For this review, use the dimensioned drawing (mm, ordinates from the lowest corner) and the shaded views. Round coordinates to 2 decimals unless told otherwise and drop trailing zeros. Order: outer loops, then holes, each group sorted by start corner. A loop starts at its lowest first (then second) coordinate and runs counter-clockwise, first axis right, second up. Notation, with made-up numbers: M 19.5,11.5 L 57.5,11.5 A30 cw 57.5,38.5 Z; hole C 38.5,5.25 d5. An arc over 180 degrees is marked long. Use a Markdown table: item, result. Add a question column.
1. Insertion check: P1, Ø12, axis at x = 32, z = 11, coming from the -Y side; P2, Ø0.9, axis at y = 1.5, z = 35.5, coming from the +X side; P3, Ø1.5, axis at y = 2, z = 6.5, coming from the -X side; P4, Ø1.5, axis at x = 9.5, y = 2, coming from the -Z side. Each pin has a flat end and moves straight along its axis. Give the tip position at first contact, or say it passes through.
2. The part is to be moulded in two halves that separate along X. For the marked faces 1, 2 and 3, say which applies: +X half, -X half, draft (parallel to the pull), parting line (faces both ways), or undercut.
3. Consider section A-A on z = 20.75. State the section outline as (x, y) points.
4. Consider section B-B on x = 20.75. State the section outline as (y, z) points, then the cut area to 3 significant figures.
5. Consider section C-C on x = 3. State the section outline as (y, z) points, then the cut area to 3 significant figures.
6. Consider section D-D on y = 0.95. Count the separate pieces of the cut face and the enclosed holes in it, then the cut area to 3 significant figures.
7. To check wall thickness, follow probe 1 along X at (y, z) = (1.9, 20.75); probe 2 along Z at (x, y) = (20.75, 1.6); probe 3 along Z at (x, y) = (38, 1). State the ranges of each line that lie inside material, in increasing order.
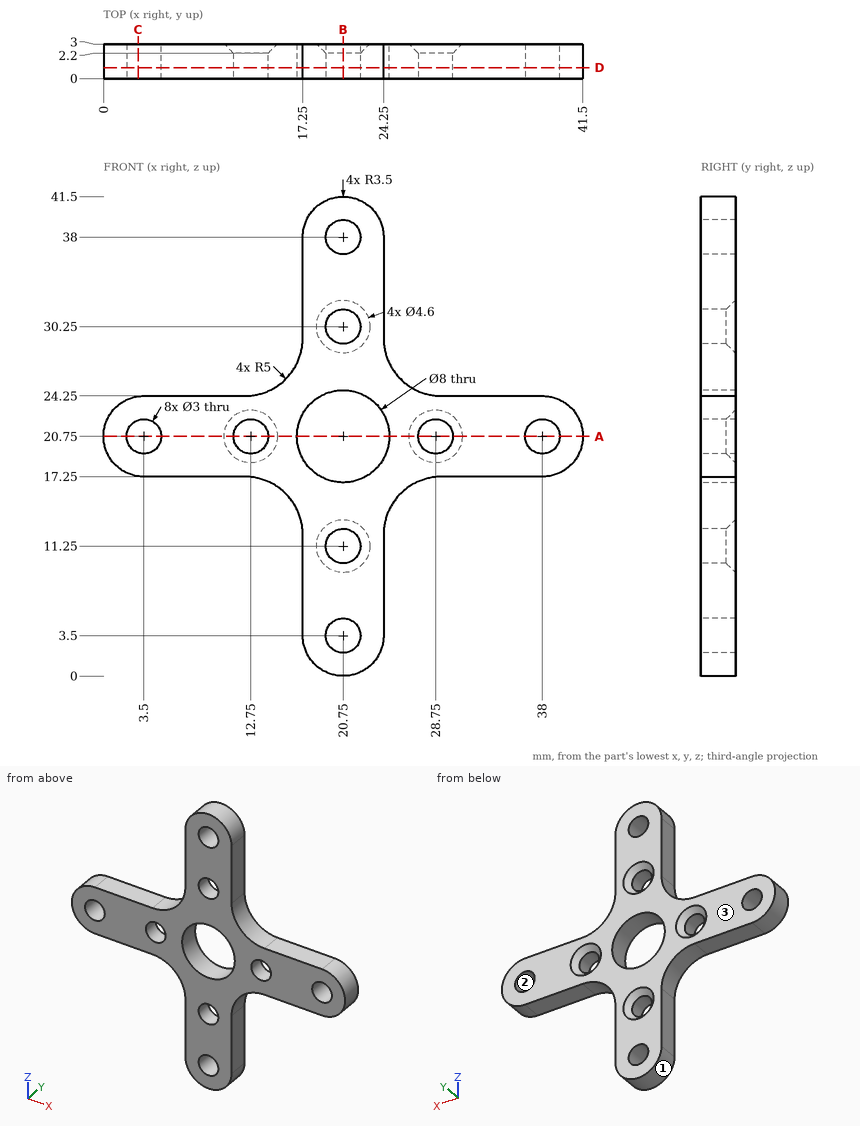
Answer block:
| question | item | result |
|---|---|---|
| 1 | P1 | through |
| 1 | P2 | x = 24.25 |
| 1 | P3 | x = 17.25 |
| 1 | P4 | z = 17.25 |
| 2 | face 1 | parting line |
| 2 | face 2 | undercut |
| 2 | face 3 | draft |
| 3 | outline | M 0,0 L 2,0 L 2,3 L 0,3 Z; M 5,0 L 11.25,0 L 11.25,2.2 L 10.45,3 L 5,3 Z; M 14.25,0 L 16.75,0 L 16.75,3 L 15.05,3 L 14.25,2.2 Z; M 24.75,0 L 27.25,0 L 27.25,2.2 L 26.45,3 L 24.75,3 Z; M 30.25,0 L 36.5,0 L 36.5,3 L 31.05,3 L 30.25,2.2 Z; M 39.5,0 L 41.5,0 L 41.5,3 L 39.5,3 Z |
| 4 | outline | M 0,0 L 3,0 L 3,2 L 0,2 Z; M 0,5 L 3,5 L 3,8.95 L 2.2,9.75 L 0,9.75 Z; M 0,12.75 L 2.2,12.75 L 3,13.55 L 3,16.75 L 0,16.75 Z; M 0,24.75 L 3,24.75 L 3,27.95 L 2.2,28.75 L 0,28.75 Z; M 0,31.75 L 2.2,31.75 L 3,32.55 L 3,36.5 L 0,36.5 Z; M 0,39.5 L 3,39.5 L 3,41.5 L 0,41.5 Z |
| 4 | area | 63.2 mm^2 |
| 5 | outline | M 0,17.29 L 3,17.29 L 3,19.34 L 0,19.34 Z; M 0,22.16 L 3,22.16 L 3,24.21 L 0,24.21 Z |
| 5 | area | 12.3 mm^2 |
| 6 | separate pieces | 1 |
| 6 | enclosed holes | 9 |
| 6 | area | 426 mm^2 |
| 7 | probe 1 | 0 to 2, 5 to 11.25, 14.25 to 16.75, 24.75 to 27.25, 30.25 to 36.5, 39.5 to 41.5 |
| 7 | probe 2 | 0 to 2, 5 to 9.75, 12.75 to 16.75, 24.75 to 28.75, 31.75 to 36.5, 39.5 to 41.5 |
| 7 | probe 3 | 17.25 to 19.25, 22.25 to 24.25 |
